Check sheet for the drawn part. Datum: minimum x, y, z corner. Units: mm. Round coordinates to 2 decimals unless told otherwise and drop trailing zeros. Loops run counter-clockwise (first coordinate to the right, second up) from the corner with the lowest first, then second, coordinate; pieces in that order, holes last. Notation, with made-up numbers: (51.25, 59) - (110.25, 59) arc R20 cw to (110.25, 84) - close; hole circle Ø10 at (-38, 17). An arc over 180 degrees is marked (long way). Use CSV: the item, a comma, the result in double quotes.
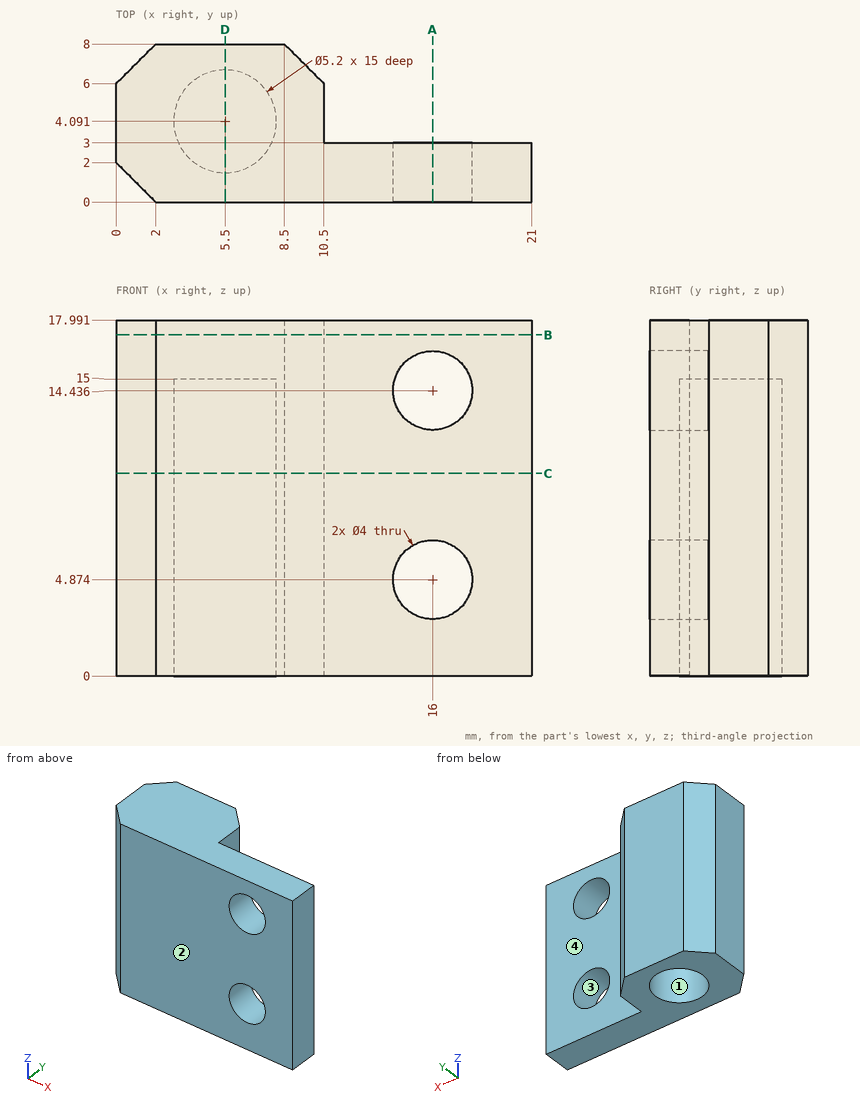
1) Cross-section at D-D, the plane x = 5.5. Record the cut outline in (y, z).
Returned:
outline,"(0, 0) - (1.49, 0) - (1.49, 15) - (6.69, 15) - (6.69, 0) - (8, 0) - (8, 17.99) - (0, 17.99) - close"
2) Gauge pin test, flat end, axial feed: pin 1 Ø2.5 at (y, z) = (5, 5) entering from +X. Record the tip position at first contact, or that the pin passes through.
Returned:
pin 1,"stops at x = 10.5"
3) Mould release check, pull along Y, two halves, no side actions. Record for the marked faces 1, 2, 3 and 4: +Y half, -Y half, draft (parallel to the pull), parting line (faces both ways), or undercut.
Returned:
face 1,"undercut"
face 2,"-Y half"
face 3,"draft"
face 4,"+Y half"
4) Cross-section at C-C, the plane z = 10.25. Record the cut outline in (x, y).
Returned:
outline,"(0, 2) - (2, 0) - (21, 0) - (21, 3) - (10.5, 3) - (10.5, 6) - (8.5, 8) - (2, 8) - (0, 6) - close; hole circle Ø5.2 at (5.5, 4.09)"
5) Thickness scan on probe 1 along Z at (x, y) = (16, 1.05); probe 2 along X at (y, z) = (2.75, 5) (1 decimal); probe 3 along Y at (x, z) = (5.5, 11.5). Record the ranges inside material, lowest first. Write a range as [from, to].
Returned:
probe 1,"z = [0, 2.87], [6.87, 12.44], [16.44, 17.99]"
probe 2,"x = [0, 3.3], [7.7, 14], [18, 21]"
probe 3,"y = [0, 1.49], [6.69, 8]"
6) Cross-section at A-A, the plane x = 16. Record the cut outline in (y, z).
Returned:
outline,"(0, 0) - (3, 0) - (3, 2.87) - (0, 2.87) - close; (0, 6.87) - (3, 6.87) - (3, 12.44) - (0, 12.44) - close; (0, 16.44) - (3, 16.44) - (3, 17.99) - (0, 17.99) - close"
7) Cross-section at B-B, the plane z = 17.25. Record the cut outline in (x, y).
Returned:
outline,"(0, 2) - (2, 0) - (21, 0) - (21, 3) - (10.5, 3) - (10.5, 6) - (8.5, 8) - (2, 8) - (0, 6) - close"
